Print and shaded views of the part. All mm, measured from the part's lowest x, y and z. Round coordinates to 2 decimals unless told otherwise and drop trailing zeros. Write each loop counter-clockwise with the first axis right and the second up, starting at its lowest first coordinate (ties: lowest second). Pieces come first, ordered by that corner, then holes.
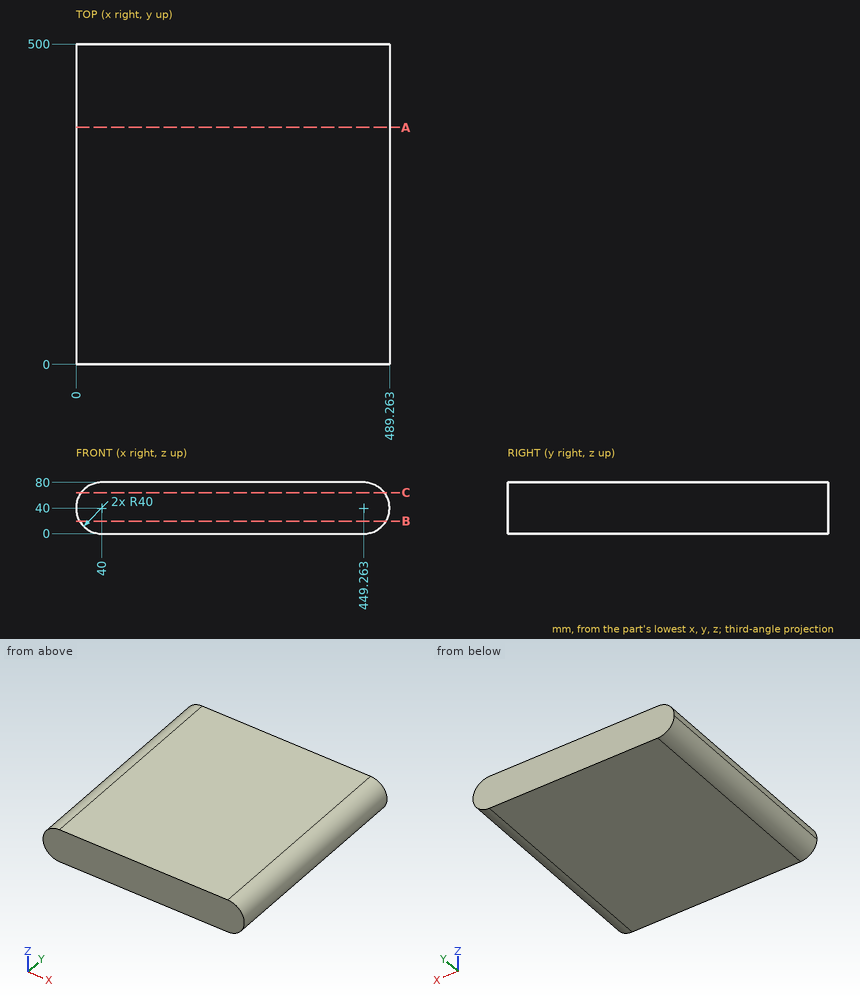
1) Slice it at A-A (y = 370). Write the cut outline in (x, z), plus the area to 3 significant figures.
Results:
outline: (40, 0) - (449.26, 0) arc R40 ccw to (449.26, 80) - (40, 80) arc R40 ccw to start
area: 37,800 mm2
2) Slice it at C-C (z = 64). Write the cut outline in (x, y).
Results:
outline: (8, 0) - (481.26, 0) - (481.26, 500) - (8, 500) - close
3) Wall check: L1, parallel to X at y = 146, z = 42; L2, parallel to X at y = 165.5, z = 17.5 (1 decimal); L3, parallel to Z at x = 467.5, y = 431. Give the ranges that are in metal, low to high.
Results:
L1: x = 0.05 to 489.21
L2: x = 6.9 to 482.3
L3: z = 4.4 to 75.6
4) Pin check, flat tips, straight feed: pin 1 Ø8 at (y, z) = (247.5, 50.5) entering from -X; pin 2 Ø2 at (x, z) = (419.5, 66) entering from -Y; pin 3 Ø8 at (y, z) = (267, 17) entering from +X; pin 4 Ø2 at (y, z) = (362, 18.5) entering from -X. Stop position of each tip, or through.
Results:
pin 1: stops at x = 0.53
pin 2: stops at y = 0
pin 3: stops at x = 484.46
pin 4: stops at x = 5.65
5) Slice it at B-B (z = 19.5). Write the cut outline in (x, y).
Results:
outline: (5.65, 0) - (483.61, 0) - (483.61, 500) - (5.65, 500) - close
